```python
from build123d import *

# Parameters (mm, degrees)
F0_R     = 1.5
F1_DEPTH = 9
F2_R     = 2.75
F3_DEPTH = 3
F5_DEPTH = 1.3
F6_SIZE  = 0.2


with BuildPart() as f1:
    # F0 (on Front) → F1 (new body)
    with BuildSketch(Plane.XZ):
        Circle(F0_R)
    extrude(amount=F1_DEPTH)

    # F2 (on face) → F3 (join)
    with BuildSketch(Plane.XZ.offset(9)):
        Circle(F2_R)
    extrude(amount=F3_DEPTH)

    # F4 (on face) → F5 (cut)
    with BuildSketch(Plane.XZ.offset(12)):
        Polygon((0.2100819211, -1.428005224), (1.3417297613, -0.5320663314), (1.1316478402, 0.8959388926), (-0.2100819211, 1.428005224), (-1.3417297613, 0.5320663314), (-1.1316478402, -0.8959388926), align=None)
    extrude(amount=-F5_DEPTH, mode=Mode.SUBTRACT)

    # F6
    f6_edges = [f1.edges().sort_by_distance(p)[0] for p in [
        (-2.75, -12, 0),
        (-2.75, -9, 0),
        (-1.5, 0, 0),
        (-1.236689, -12, -0.181936),
        (-0.460783, -12, -1.161972),
        (0.775906, -12, -0.980036),
        (1.236689, -12, 0.181936),
        (0.460783, -12, 1.161972),
        (-0.775906, -12, 0.980036),
    ]]
    chamfer(f6_edges, length=F6_SIZE)


solid = f1.part
```
Geometry check sheet. Reference: the model listing, model coordinates, mm. A direction names the side the tool comes from. Coordinates: 2 decimals unless noted, no trailing zeros. Write each loop counter-clockwise with the first axis right and the second up, starting at its lowest first coordinate (ties: lowest second). Pieces come first, ordered by that corner, then holes. Notation, with made-up numbers: M 61.5,22.5 L 92.5,22.5 A16 cw 92.5,27.5 Z; hole C 68,46.25 d9. An arc over 180 degrees is marked long. Use one line per item in the form item = value. Start each with the question number.
1) Thickness scan on probe 1 along X at (y, z) = (-11.5, 2.35); probe 2 along Z at (x, y) = (-0.1, -9.5); probe 3 along Y at (x, z) = (-1.5, -1.4). Record the ranges inside material, lowest first. Write a range as from..to.
2) Section check A-A on z = 0. Enter the section's corners in (x, y).
3) Set-up check for faces 1 (the flat face through (0, -12, -2)), 2 (the flat face through (0, -10.7, 0)), 3 (the flat face through (0, -9, -2)): record each of +Z, -Z, +X, -X, +Y, -Y from which the full face is reachable in a straight line by a thin tool's end or side.
4) Section check C-C on y = -10. Enter the section's corners in (x, z), and give its area (3 significant figures).
5) Go/stop test with flat-tipped pins: pin 1 Ø3 at (y, z) = (-4, 1) entering from +X; pin 2 Ø0.8 at (x, z) = (-0.5, -0.5) entering from -Y; pin 3 Ø3 at (y, z) = (-6, -1.5) entering from -X. Record where each tip stops, or that it passes through.
6) Section check B-B on x = 0. Enter the section's corners in (y, z), and give its area (3 significant figures).
7) Section check D-D on y = -4. Enter the section's corners in (x, z).
8) Release check for a two-part mould opening along X. For faces 4 (the flat face through (0.47, -11.26, 1.16)), 5 (the flat face through (0, 0, 0)), 6 (the cylindrical face through (-1.5, -4.54, 0.07)) record: pulls with the +X half, pulls with the -X half, needs draft (parallel to the pull), parting line crosses it, or undercut.
Responses:
q1.probe_1 = -1.43..1.43
q1.probe_2 = -2.75..2.75
q1.probe_3 = -12..-9
q2.outline = M -2.75,-11.8 L -2.55,-12 L -1.47,-12 L -1.26,-11.8 L -1.26,-10.7 L 1.26,-10.7 L 1.26,-11.8 L 1.47,-12 L 2.55,-12 L 2.75,-11.8 L 2.75,-9.2 L 2.55,-9 L 1.5,-9 L 1.5,-0.2 L 1.3,0 L -1.3,0 L -1.5,-0.2 L -1.5,-9 L -2.55,-9 L -2.75,-9.2 Z
q3.face_1 = +Z, -Z, +X, -X, -Y
q3.face_2 = -Y
q3.face_3 = +Y
q4.outline = C 0,0 d5.5
q4.area = 23.8 mm2
q5.pin_1 = 1.5
q5.pin_2 = -10.7
q5.pin_3 = -1.5
q6.outline = M -12,-2.55 L -11.8,-2.75 L -9.2,-2.75 L -9,-2.55 L -9,-1.5 L -0.2,-1.5 L 0,-1.3 L 0,1.3 L -0.2,1.5 L -9,1.5 L -9,2.55 L -9.2,2.75 L -11.8,2.75 L -12,2.55 L -12,1.56 L -11.8,1.34 L -10.7,1.34 L -10.7,-1.34 L -11.8,-1.34 L -12,-1.56 Z
q6.area = 39.8 mm2
q7.outline = C 0,0 d3
q8.face_4 = undercut
q8.face_5 = needs draft
q8.face_6 = parting line crosses it
